Check sheet for the modelled part. Datum: model origin and axes. Units: mm. A direction names the side the tool comes from. Round coordinates to 2 decimals unless told otherwise and drop trailing zeros. Loops run counter-clockwise (first coordinate to the right, second up) from the corner with the lowest first, then second, coordinate; pieces in that order, holes last. Notation, with made-up numbers: (-32.5, 76) - (20.5, 76) arc R22 cw to (20.5, 112) - close; hole circle Ø3 at (50, 16.5). An arc over 180 degrees is marked (long way). Return JSON: item names as keys, results as strings.
from build123d import *

# Parameters (mm, degrees)
F0_W     = 101.6
F0_H     = 57.15
F1_DEPTH = 3.175
F2_W     = 12.7
F2_H     = 3.175
F2_W_2   = 3.175
F2_H_2   = 12.7
F3_DEPTH = 3.176
F5_D     = 3.556


with BuildPart() as f1:
    # F0 (on Top) → F1 (new body)
    with BuildSketch(Plane.XY):
        Rectangle(F0_W, F0_H)
    extrude(amount=F1_DEPTH)

    # F2 (on face) → F3 (cut, through all)
    with BuildSketch(Plane.XY.offset(3.175)):
        with Locations((-25.4, -26.9875)):
            Rectangle(F2_W, F2_H)
        with Locations((0, -26.9875)):
            Rectangle(F2_W, F2_H)
        with Locations((25.4, -26.9875)):
            Rectangle(F2_W, F2_H)
        with Locations((44.1325, -12.065)):
            Rectangle(F2_W_2, F2_H_2)
        with Locations((44.1325, 12.065)):
            Rectangle(F2_W_2, F2_H_2)
        with Locations((-25.4, 26.9875)):
            Rectangle(F2_W, F2_H)
        with Locations((0, 26.9875)):
            Rectangle(F2_W, F2_H)
        with Locations((25.4, 26.9875)):
            Rectangle(F2_W, F2_H)
    extrude(amount=-F3_DEPTH, mode=Mode.SUBTRACT)

    # F5 (through all)
    with Locations(Plane(origin=(0, 0, 0), x_dir=(1, 0, 0), z_dir=(0, 0, -1))):
        with Locations((-12.566888, 26.543), (12.935686, 26.543), (-12.566888, -26.543), (12.935686, -26.543)):
            Hole(F5_D / 2)


solid = f1.part
Q1. Sectioned sample at B-B (x = 2). Enter the section's corners in (y, z) (3 decimals).
Answer key:
{"outline": "(-25.4, 0) - (25.4, 0) - (25.4, 3.175) - (-25.4, 3.175) - close"}
Q2. Tool access check on faces 4 (the face through (25, -25.4, 2)), 5 (the face through (45.72, 12, 2)), 6 (the face through (-19.05, 27, 2)). Record the directions out of +Z, -Z, +X, -X, +Y, -Y that give a thin tool (end or side, any length) a straight path to the whole face; none if there is none.
Answer key:
{"face 4": "+Z, -Z, -Y", "face 5": "+Z, -Z", "face 6": "+Z, -Z, +Y"}
Q3. Depth check by flat-ended pin: P1, Ø1.6, axis at x = -27, z = 2, coming from the -Y side; P2, Ø3, axis at x = 12.94, y = 26.54, coming from the -Z side. Enter the tip coordinate at first touch or a pass-through.
Answer key:
{"P1": "stops at y = -25.4", "P2": "passes through"}
Q4. Draft check along X on faces 1 (the face through (50.8, 0, 2)), 2 (the face through (-1, 0, 0)), 3 (the face through (6.35, -27, 2)). Enter one of: released by +X, released by -X, zero draft, split by the parting line, or undercut.
Answer key:
{"face 1": "released by +X", "face 2": "zero draft", "face 3": "undercut"}
Q5. Scan lines: probe 1 along Y at (x, z) = (13, 1.85) (3 decimals); probe 2 along X at (y, z) = (-9.5, 2.9) (3 decimals); probe 3 along Y at (x, z) = (14.5, 1.1) (3 decimals). Record each from-to range of solid material in increasing order. Write a range as [from, to].
Answer key:
{"probe 1": "y = [-28.575, -28.32], [-24.766, 24.766], [28.32, 28.575]", "probe 2": "x = [-50.8, 42.545], [45.72, 50.8]", "probe 3": "y = [-28.575, -27.388], [-25.698, 25.698], [27.388, 28.575]"}
Q6. Sectioned sample at A-A (y = 10). Enter the section's corners in (x, z) (3 decimals), plus the area to 4 significant figures.
Answer key:
{"outline": "(-50.8, 0) - (42.545, 0) - (42.545, 3.175) - (-50.8, 3.175) - close; (45.72, 0) - (50.8, 0) - (50.8, 3.175) - (45.72, 3.175) - close", "area": "312.5 mm²"}
Q7. Sectioned sample at C-C (z = 0.55). State how many separate pieces and enclosed holes the cut face has, plus the area to 3 significant figures.
Answer key:
{"separate pieces": "1", "enclosed holes": "6", "area": "5,440 mm²"}
